Geometry: final body of the model. Coordinates: model frame, mm. A direction names the side the tool comes from. Give positions to 0.01 mm unless a question says otherwise; leave off trailing zeros. Write each loop counter-clockwise with the first axis right and the second up, starting at its lowest first coordinate (ties: lowest second). Pieces come first, ordered by that corner, then holes.
```python
from build123d import *

# Parameters (mm, degrees)
CROQUIS2_W              = 75
CROQUIS2_H              = 75
SALIENTE_EXTRUIR1_DEPTH = 5
SALIENTE_EXTRUIR2_DEPTH = 100
CHAFL_N1_SIZE           = 25
CHAFL_N1_SIZE_2         = 15
CHAFL_N2_SIZE           = 25
CHAFL_N2_SIZE_2         = 15
CORTAR_EXTRUIR1_REACH   = 112.598
CHAFL_N3_SIZE           = 5
REDONDEO1_R             = 6
REDONDEO2_R             = 20
SKETCH1_R               = 4.15
CUT_EXTRUDE2_DEPTH      = 10


with BuildPart() as part:
    # Croquis2 → Saliente-Extruir1 (new body)
    with BuildSketch(Plane(origin=(0, 0, 0), x_dir=(0, 1, 0), z_dir=(0, 0, 1))):
        Rectangle(CROQUIS2_W, CROQUIS2_H)
    extrude(amount=SALIENTE_EXTRUIR1_DEPTH)

    # Croquis2<3> → Saliente-Extruir2 (add)
    with BuildSketch(Plane(origin=(0, 0, 0), x_dir=(0, 1, 0), z_dir=(0, 0, 1))):
        with BuildLine():
            Line((-21.5, 9.375), (-21.5, -9.375))
            Line((-21.5, -9.375), (-8.267972847, -9.375))
            ThreePointArc((-8.267972847, -9.375), (-12.5, 0), (-8.267972847, 9.375))
            Line((-8.267972847, 9.375), (-21.5, 9.375))
        make_face()
        with BuildLine():
            ThreePointArc((8.267972847, 9.375), (12.5, 0), (8.267972847, -9.375))
            Line((8.267972847, -9.375), (21.5, -9.375))
            Line((21.5, -9.375), (21.5, 9.375))
            Line((21.5, 9.375), (8.267972847, 9.375))
        make_face()
    extrude(amount=-SALIENTE_EXTRUIR2_DEPTH)

    # Chaflán1
    # the kernel refuses this chamfer: 25, 15 mm, written as the material it takes off along each edge
    with BuildSketch(Plane(origin=(74.03152743, 21.5, -100), x_dir=(0, 0.01989341895858247, 0.9998021063601227), z_dir=(-1, 0, 0))) as chafl_n1_piece_1:
        Polygon((CHAFL_N1_SIZE * 0.99980210636, -CHAFL_N1_SIZE * 0.0198934189586), (-CHAFL_N1_SIZE_2 * 0.0198934189586, -CHAFL_N1_SIZE_2 * 0.99980210636), (0, 0), align=None)
    extrude(amount=148.06305486, mode=Mode.SUBTRACT)

    # Chaflán2
    # the kernel refuses this chamfer: 25, 15 mm, written as the material it takes off along each edge
    with BuildSketch(Plane(origin=(-74.03152743, -21.5, -100), x_dir=(0, -0.01989341895858247, 0.9998021063601227), z_dir=(1, 0, 0))) as chafl_n2_piece_1:
        Polygon((CHAFL_N2_SIZE * 0.99980210636, -CHAFL_N2_SIZE * 0.0198934189586), (-CHAFL_N2_SIZE_2 * 0.0198934189586, -CHAFL_N2_SIZE_2 * 0.99980210636), (0, 0), align=None)
    extrude(amount=148.06305486, mode=Mode.SUBTRACT)

    # Croquis2<4> → Cortar-Extruir1 (cut, up to next)
    with BuildSketch(Plane(origin=(0, 0, 0), x_dir=(0, 1, 0), z_dir=(0, 0, 1)), mode=Mode.PRIVATE) as cortar_extruir1_sk1:
        with BuildLine():
            ThreePointArc((-8.267972847, 9.375), (-12.5, 0), (-8.267972847, -9.375))
            Line((-8.267972847, -9.375), (8.267972847, -9.375))
            ThreePointArc((8.267972847, -9.375), (11.392972847, -5.142972847), (12.5, 0))
            ThreePointArc((12.5, 0), (11.392972847, 5.142972847), (8.267972847, 9.375))
            Line((8.267972847, 9.375), (-8.267972847, 9.375))
        make_face()
    cortar_extruir1_tool1 = extrude(cortar_extruir1_sk1.sketch, amount=CORTAR_EXTRUIR1_REACH, mode=Mode.PRIVATE) & part.part
    # Croquis2<4> → Cortar-Extruir1 (cut, up to next)
    with BuildSketch(Plane(origin=(0, 0, 0), x_dir=(0, 1, 0), z_dir=(0, 0, 1)), mode=Mode.PRIVATE) as cortar_extruir1_sk2:
        with BuildLine():
            Line((8.267972847, -9.375), (-8.267972847, -9.375))
            ThreePointArc((-8.267972847, -9.375), (0, -12.5), (8.267972847, -9.375))
        make_face()
    cortar_extruir1_tool2 = extrude(cortar_extruir1_sk2.sketch, amount=CORTAR_EXTRUIR1_REACH, mode=Mode.PRIVATE) & part.part
    # Croquis2<4> → Cortar-Extruir1 (cut, up to next)
    with BuildSketch(Plane(origin=(0, 0, 0), x_dir=(0, 1, 0), z_dir=(0, 0, 1)), mode=Mode.PRIVATE) as cortar_extruir1_sk3:
        with BuildLine():
            ThreePointArc((8.267972847, 9.375), (0, 12.5), (-8.267972847, 9.375))
            Line((-8.267972847, 9.375), (8.267972847, 9.375))
        make_face()
    cortar_extruir1_tool3 = extrude(cortar_extruir1_sk3.sketch, amount=CORTAR_EXTRUIR1_REACH, mode=Mode.PRIVATE) & part.part
    add(cortar_extruir1_tool1.solids().sort_by_distance((0, 0, 0))[0], mode=Mode.SUBTRACT)
    add(cortar_extruir1_tool2.solids().sort_by_distance((10.639442, 0, 0))[0], mode=Mode.SUBTRACT)
    add(cortar_extruir1_tool3.solids().sort_by_distance((-10.639442, 0, 0))[0], mode=Mode.SUBTRACT)

    # Chaflán3
    chafl_n3_edges = [part.edges().sort_by_distance(p)[0] for p in [
        (0, 21.5, -75),
        (0, -21.5, -75),
    ]]
    chamfer(chafl_n3_edges, length=CHAFL_N3_SIZE)

    # Redondeo1
    redondeo1_edges = [part.edges().sort_by_distance(p)[0] for p in [
        (-9.375, -21.5, -35),
        (9.375, -21.5, -35),
        (9.375, 21.5, -35),
        (-9.375, 21.5, -35),
    ]]
    fillet(redondeo1_edges, radius=REDONDEO1_R)

    # Redondeo2
    redondeo2_edges = [part.edges().sort_by_distance(p)[0] for p in [
        (37.5, 37.5, 2.5),
        (37.5, -37.5, 2.5),
        (-37.5, -37.5, 2.5),
        (-37.5, 37.5, 2.5),
    ]]
    fillet(redondeo2_edges, radius=REDONDEO2_R)

    # Sketch1 → Cut-Extrude2 (cut)
    with BuildSketch(Plane.XY.offset(5)):
        with Locations((25.5, 19.5)):
            Circle(SKETCH1_R)
        with Locations((-24.48, 24.48)):
            Circle(SKETCH1_R)
        with Locations((-25.5, -19.5)):
            Circle(SKETCH1_R)
    extrude(amount=-CUT_EXTRUDE2_DEPTH, mode=Mode.SUBTRACT)


solid = part.part
```
Item 1: Section C-C, the plane y = -9.5. Return the cut outline in (x, z) (3 decimals), plus the area to 3 significant figures.
Found:
outline: (-37.5, 0) - (-9.375, 0) - (-9.375, -95) - (-8.124, -95) - (-8.124, 5) - (-37.5, 5) - close; (8.124, -95) - (9.375, -95) - (9.375, 0) - (37.5, 0) - (37.5, 5) - (8.124, 5) - close
area: 531 mm2
Item 2: Line query: L1, parallel to Y at x = -25, z = 3; L2, parallel to Z at x = 22, y = 32.5; L3, parallel to Y at x = 4, z = -44.5. Output: solid intervals per line, ascending.
Found:
L1: y = -36.04 to -23.62, -15.38 to 20.36, 28.6 to 36.04
L2: z = 0 to 5
L3: y = -21.47 to -11.84, 11.84 to 21.47
Item 3: Pin query (flat end, axial travel): pin 1 Ø9.5 at (x, y) = (25.5, 19.5) entering from -Z; pin 2 Ø6 at (x, y) = (-4.5, -14) entering from -Z; pin 3 Ø6 at (x, z) = (0, -55) entering from -Y; pin 4 Ø7.5 at (x, y) = (-24.48, 24.48) entering from +Z. Return the tip coordinate at first contact, or that it passes through.
Found:
pin 1: stops at z = 0
pin 2: stops at z = -92.18
pin 3: stops at y = -21.5
pin 4: passes through
Item 4: Section A-A, the plane z = -18. Return the cut outline in (x, y) (3 decimals), plus the area to 3 significant figures.
Found:
outline: (-9.375, -15.5) arc R6 ccw to (-3.375, -21.5) - (3.375, -21.5) arc R6 ccw to (9.375, -15.5) - (9.375, -8.268) arc R12.5 cw to (-9.375, -8.268) - close; (-9.375, 8.268) arc R12.5 cw to (9.375, 8.268) - (9.375, 15.5) arc R6 ccw to (3.375, 21.5) - (-3.375, 21.5) arc R6 ccw to (-9.375, 15.5) - close
area: 355 mm2
Item 5: Pull-direction query (X, two-part tool) for faces 1 (the face through (-26.4, -23.55, 2.54)), 2 (the face through (7.57, -19.79, -43.1)), 3 (the face through (0, -21.5, -35)), 4 (the face through (24.6, 15.45, 2.54)); classes: +X half, -X half, draft (parallel to the pull), parting line (faces both ways), or undercut.
Found:
face 1: undercut
face 2: +X half
face 3: draft
face 4: undercut
Item 6: Section B-B, the plane x = -25.5. Return the cut outline in (y, z).
Found:
outline: (-35.83, 0) - (-23.65, 0) - (-23.65, 5) - (-35.83, 5) - close; (-15.35, 0) - (20.46, 0) - (20.46, 5) - (-15.35, 5) - close; (28.5, 0) - (35.83, 0) - (35.83, 5) - (28.5, 5) - close
Item 7: Section D-D, the plane z = -88.5. Return the cut outline in (x, y) (3 decimals).
Found:
outline: (-9.375, -13.4) - (9.375, -13.4) - (9.375, -8.268) arc R12.5 cw to (-9.375, -8.268) - close; (-9.375, 8.268) arc R12.5 cw to (9.375, 8.268) - (9.375, 13.4) - (-9.375, 13.4) - close
Item 8: Reachability of faces 5 (the face through (-7.57, 19.79, -43.1)), 6 (the face through (-9, -9, 5)), 7 (the face through (9.375, -12, -48)), 8 (the face through (-7.57, -19.79, -43.1)), 9 (the face through (-9.375, 12, -48)) from +Z, -Z, +X, -X, +Y, -Y: full face, straight path, thin tool, end or side. Return the list, or none.
Found:
face 5: -Z, -X, +Y
face 6: +Z, +X, -X, +Y, -Y
face 7: -Z, +X, +Y, -Y
face 8: -Z, -X, -Y
face 9: -Z, -X, +Y, -Y
